Build history of the part. All positions in model axes, mm. Face numbers are marked on the shaded views. Round coordinates to 2 decimals unless told otherwise and drop trailing zeros. Write each loop counter-clockwise with the first axis right and the second up, starting at its lowest first coordinate (ties: lowest second). Pieces come first, ordered by that corner, then holes. Notation, with made-up numbers: (-28, 60.5) - (29, 60.5) arc R11 cw to (29, 66.5) - close; hole circle Ø9 at (-21.5, -39.5). An arc over 180 degrees is marked (long way). Answer as a JSON object with one key per item and string values. Group by question number.
Item 1: Slice it at B-B, the plane x = -19. List the corners of the cut face in (y, z).
Item 2: Flat gauge pins, fed straight in: pin 1 (1 mm diameter, centred on x = 3, z = 2.5, fed in from -Y); pin 2 (1 mm diameter, centred on x = 1.5, y = 49.5, fed in from -Z); pin 3 (1 mm diameter, centred on y = 91.5, z = -4.5, fed in from -X); pin 4 (1.6 mm diameter, centred on y = 219, z = 3, fed in from +X). Where does each tip first touch, or does it go through?
Item 3: Two-plate mould, pull along X, no slides. Class the marked faces 1 and 2: +X half, -X half, draft (parallel to the pull), parting line (faces both ways), or undercut.
Item 4: Slice it at A-A, the plane y = 246.25. List the corners of the cut face in (x, z).
Item 5: Probe line 1 (Y direction, x = 1, z = 2.5); line 2 (Z direction, x = 15.5, y = 36); line 3 (X direction, y = 365, z = 3). List the from-to ranges inside material, lowest first. Write a range as from..to.
from build123d import *

# Parameters (mm, degrees)
SKETCH_11_W             = 80.498191281
SKETCH_11_H             = 375
SM_BASE_FLANGE_1_DEPTH  = 2
CUT_EXTRUDE_1_DEPTH     = 378.392627604
HOLE_WIZARD_3_0_3_1_D   = 3
HOLE_WIZARD_3_0_3_2_D   = 3
HOLE_WIZARD_13_0_13_1_D = 13
OTHER_1_DEPTH           = 375
OTHER_1_2_DEPTH         = 375
OTHER_START             = -25
OTHER_1_3_OUTLINE_R     = 1.5
OTHER_1_3_DEPTH         = 4
OTHER_START_2           = 33.158957521
OTHER_3_OUTLINE_R       = 1.5
OTHER_3_DEPTH           = 6.841042479
OTHER_3_2_DEPTH         = 375
OTHER_3_3_DEPTH         = 375
OTHER_START_3           = 24
OTHER_3_4_OUTLINE_R     = 1.5
OTHER_3_4_DEPTH         = 4


with BuildPart() as part:
    # 基材-凸緣1: sheet metal written as solids
    # 草圖11 → 基材-凸緣1 (new body)
    with BuildSketch(Plane.XY.offset(4)):
        with Locations((2.132449513, 187.5)):
            Rectangle(SKETCH_11_W, SKETCH_11_H)
    extrude(amount=-SM_BASE_FLANGE_1_DEPTH)

    # 草圖16 → 除料-伸長1 (cut, through all)
    with BuildSketch(Plane(origin=(0, 0, 2), x_dir=(-1, 0, 0), z_dir=(0, 0, -1))):
        with BuildLine():
            Line((1.517550486, 220.75), (-5.782449514, 220.75))
            ThreePointArc((-5.782449514, 220.75), (-6.489556295, 220.457106781), (-6.782449514, 219.75))
            Line((-6.782449514, 219.75), (-6.782449514, 218.25))
            ThreePointArc((-6.782449514, 218.25), (-6.489556295, 217.542893219), (-5.782449514, 217.25))
            Line((-5.782449514, 217.25), (1.517550486, 217.25))
            ThreePointArc((1.517550486, 217.25), (2.224657268, 217.542893219), (2.517550486, 218.25))
            Line((2.517550486, 218.25), (2.517550486, 219.75))
            ThreePointArc((2.517550486, 219.75), (2.224657268, 220.457106781), (1.517550486, 220.75))
        make_face()
    extrude(amount=-CUT_EXTRUDE_1_DEPTH, mode=Mode.SUBTRACT)

    # Ø3.0 (3) 直徑孔1 (through all)
    with Locations(Plane.XY.offset(4)):
        with Locations((37.381545154, 70), (37.381545154, 187.5), (37.381545154, 305), (-33.116646127, 70), (-33.116646127, 187.5), (-33.116646127, 305)):
            Hole(HOLE_WIZARD_3_0_3_1_D / 2)

    # Ø3.0 (3) 直徑孔2 (through all)
    with Locations(Plane(origin=(0, 0, 2), x_dir=(-1, 0, 0), z_dir=(0, 0, -1))):
        with Locations((-12.882449514, 219), (8.617550486, 219), (5.367550486, 10), (-9.632449514, 10), (-9.632449514, 365), (5.367550486, 365)):
            Hole(HOLE_WIZARD_3_0_3_2_D / 2)

    # Ø13.0 (13) 直徑孔1 (through all)
    with Locations(Plane.XY.offset(4)):
        with Locations((2.132449514, 246.25)):
            Hole(HOLE_WIZARD_13_0_13_1_D / 2)

    # Other 1: read off the stored shape, not the designer's step
    # Other 1 outline → Other 1 (cut)
    with BuildSketch(Plane(origin=(0, 0, 0), x_dir=(1, 0, 0), z_dir=(0, 1, 0))):
        with BuildLine():
            Line((-26.042976967, -2.5), (-26.331652102, -2))
            Line((-26.331652102, -2), (-38.116646127, -2))
            Line((-38.116646127, -2), (-38.116646127, -4))
            Line((-38.116646127, -4), (-23.444900756, -4))
            ThreePointArc((-23.444900756, -4), (-24.944900756, -3.598076211), (-26.042976967, -2.5))
        make_face()
    extrude(amount=OTHER_1_DEPTH, mode=Mode.SUBTRACT)

    # Other 1 2 outline → Other 1 2 (add)
    with BuildSketch(Plane(origin=(0, 0, 0), x_dir=(1, 0, 0), z_dir=(0, 1, 0))):
        with BuildLine():
            Line((-30.599601294, 9.392304845), (-32.331652102, 8.392304845))
            Line((-32.331652102, 8.392304845), (-26.331652102, -2))
            Line((-26.331652102, -2), (-23.444900756, -2))
            ThreePointArc((-23.444900756, -2), (-23.944900756, -1.866025404), (-24.310926159, -1.5))
            Line((-24.310926159, -1.5), (-30.599601294, 9.392304845))
        make_face()
    extrude(amount=OTHER_1_2_DEPTH)

    # Other 1 3 outline → Other 1 3 (cut)
    with BuildSketch(Plane(origin=(0, 0, 0), x_dir=(0.4999999999999988, 0, 0.8660254037844395), z_dir=(0.8660254037844393, 0, -0.4999999999999991)).offset(OTHER_START)):
        with Locations((-18.433775243, -305)):
            Circle(OTHER_1_3_OUTLINE_R)
        with Locations((-18.433775243, -187.5)):
            Circle(OTHER_1_3_OUTLINE_R)
        with Locations((-18.433775243, -70)):
            Circle(OTHER_1_3_OUTLINE_R)
    extrude(amount=OTHER_1_3_DEPTH, mode=Mode.SUBTRACT)

    # Other 3: read off the stored shape, not the designer's step
    # Other 3 outline → Other 3 (cut)
    with BuildSketch(Plane(origin=(0, 0, 0), x_dir=(0.500000000000006, 0, -0.8660254037844353), z_dir=(0.8660254037844352, 0, 0.5000000000000061)).offset(OTHER_START_2)):
        with Locations((20.566224757, 70)):
            Circle(OTHER_3_OUTLINE_R)
        with Locations((20.566224757, 187.5)):
            Circle(OTHER_3_OUTLINE_R)
        with Locations((20.566224757, 305)):
            Circle(OTHER_3_OUTLINE_R)
    extrude(amount=OTHER_3_DEPTH, mode=Mode.SUBTRACT)

    # Other 3 2 outline → Other 3 2 (cut)
    with BuildSketch(Plane(origin=(0, 0, 0), x_dir=(1, 0, 0), z_dir=(0, 1, 0))):
        with BuildLine():
            Line((42.381545154, -2), (30.596551129, -2))
            Line((30.596551129, -2), (30.307875994, -2.5))
            ThreePointArc((30.307875994, -2.5), (29.209799783, -3.598076211), (27.709799783, -4))
            Line((27.709799783, -4), (42.381545154, -4))
            Line((42.381545154, -4), (42.381545154, -2))
        make_face()
    extrude(amount=OTHER_3_2_DEPTH, mode=Mode.SUBTRACT)

    # Other 3 3 outline → Other 3 3 (add)
    with BuildSketch(Plane(origin=(0, 0, 0), x_dir=(1, 0, 0), z_dir=(0, 1, 0))):
        with BuildLine():
            Line((34.864500321, 9.392304845), (28.575825186, -1.5))
            ThreePointArc((28.575825186, -1.5), (28.209799783, -1.866025404), (27.709799783, -2))
            Line((27.709799783, -2), (30.596551129, -2))
            Line((30.596551129, -2), (36.596551129, 8.392304845))
            Line((36.596551129, 8.392304845), (34.864500321, 9.392304845))
        make_face()
    extrude(amount=OTHER_3_3_DEPTH)

    # Other 3 4 outline → Other 3 4 (cut)
    with BuildSketch(Plane(origin=(0, 0, 0), x_dir=(0.500000000000006, 0, -0.8660254037844353), z_dir=(0.8660254037844352, 0, 0.5000000000000061)).offset(OTHER_START_3)):
        with Locations((20.566224757, 70)):
            Circle(OTHER_3_4_OUTLINE_R)
        with Locations((20.566224757, 187.5)):
            Circle(OTHER_3_4_OUTLINE_R)
        with Locations((20.566224757, 305)):
            Circle(OTHER_3_4_OUTLINE_R)
    extrude(amount=OTHER_3_4_DEPTH, mode=Mode.SUBTRACT)


solid = part.part
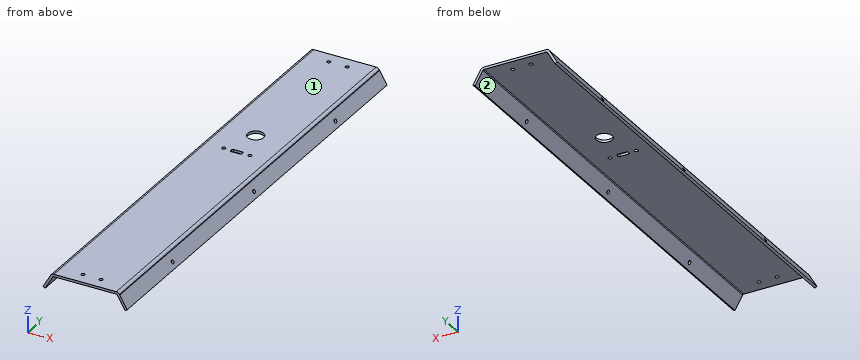
Geometry says:
{
 "1": {"outline": "(0, 2) - (375, 2) - (375, 4) - (0, 4) - close"},
 "2": {"pin 1": "stops at y = 0", "pin 2": "stops at z = 2", "pin 3": "stops at x = -30.37", "pin 4": "stops at x = 30.48"},
 "3": {"face 1": "draft", "face 2": "undercut"},
 "4": {"outline": "(-32.33, -8.39) - (-30.6, -9.39) - (-24.31, 1.5) arc R1 cw to (-23.44, 2) - (-4.37, 2) - (-4.37, 4) - (-23.44, 4) arc R3 ccw to (-26.04, 2.5) - close; (8.63, 2) - (27.71, 2) arc R1 cw to (28.58, 1.5) - (34.86, -9.39) - (36.6, -8.39) - (30.31, 2.5) arc R3 ccw to (27.71, 4) - (8.63, 4) - close"},
 "5": {"line 1": "y = 0..217.25, 220.75..239.85, 252.65..375", "line 2": "z = 2..4", "line 3": "x = -25.68..-6.87, -3.87..8.13, 11.13..29.95"}
}
